```python
from build123d import *

# Parameters (mm, degrees)
F0_W     = 22.5599961265
F0_H     = 4
F1_DEPTH = 150
F2_R     = 2
F3_DEPTH = 9.20100235
F4_SIZE  = 1


# Not quite as in the source:
# - a fillet or chamfer that OpenCascade refuses, or shapes differently, is made with other operations: its cross-section is extruded or revolved along the edge and cut away or added


with BuildPart() as f1:
    # F0 (on Top) → F1 (new body)
    with BuildSketch(Plane.XY):
        Polygon((0, -4), (0, 0), (-8.7200025445, -5.20000235), (-20.5118006432, -5.20000235), (-27.4400038735, -9.20000235), (-8.7200025445, -9.20000235), align=None)
        with Locations((11.2799980633, -2)):
            Rectangle(F0_W, F0_H)
        with Locations((33.8399941898, -2)):
            Rectangle(F0_W, F0_H)
        Polygon((53.8399947975, -5.20000235), (45.119992253, 0), (45.119992253, -4), (53.8399947975, -9.20000235), (72.5599961265, -9.20000235), (65.6317928962, -5.20000235), align=None)
    extrude(amount=F1_DEPTH)

    # F2 (on face) → F3 (cut, through all)
    with BuildSketch(Plane.XZ.offset(9.20000235)):
        with Locations((-14.9400038735, 140)):
            Circle(F2_R)
        with Locations((60.0599961265, 140)):
            Circle(F2_R)
        with Locations((-14.9400038735, 10)):
            Circle(F2_R)
        with Locations((60.0599961265, 10)):
            Circle(F2_R)
    extrude(amount=-F3_DEPTH, mode=Mode.SUBTRACT)

    # F4
    f4_edges = [f1.edges().sort_by_distance(p)[0] for p in [
        (58.059996, -5.200002, 140),
    ]]
    chamfer(f4_edges, length=F4_SIZE)

    # F5: chamfer of 2 on 1 edges, made by hand

    # F5_s1 → F5_t2 (revolve, cut)
    with BuildSketch(Plane.XY.offset(140)):
        Polygon((63.4742096889, -4.7857887876), (62.0599961265, -8.20000235), (62.0599961265, -6.20000235), align=None)
    revolve(axis=Axis((60.0599961265, -6.20000235, 140), (0, -1, 0)), mode=Mode.SUBTRACT)

    # F6: chamfer of 1.5 on 4 edges, made by hand

    # F6_s1 → F6_t2 (revolve, cut)
    with BuildSketch(Plane.XY.offset(10)):
        Polygon((63.5599961265, -5.20000235), (62.0599961265, -6.70000235), (62.0599961265, -5.20000235), align=None)
    revolve(axis=Axis((60.0599961265, -5.20000235, 10), (0, -1, 0)), mode=Mode.SUBTRACT)

    # F6_s3 → F6_t4 (revolve, cut)
    with BuildSketch(Plane.XY.offset(10)):
        Polygon((-11.4400038735, -5.20000235), (-12.9400038735, -6.70000235), (-12.9400038735, -5.20000235), align=None)
    revolve(axis=Axis((-14.9400038735, -5.20000235, 10), (0, -1, 0)), mode=Mode.SUBTRACT)

    # F6_s5 → F6_t6 (revolve, cut)
    with BuildSketch(Plane.XY.offset(140)):
        Polygon((-11.4400038735, -5.20000235), (-12.9400038735, -6.70000235), (-12.9400038735, -5.20000235), align=None)
    revolve(axis=Axis((-14.9400038735, -5.20000235, 140), (0, -1, 0)), mode=Mode.SUBTRACT)

    # F6_s7 → F6_t8 (revolve, cut)
    with BuildSketch(Plane.XY.offset(140)):
        Polygon((62.1741768278, -7.9243457525), (62.0599961265, -8.498370901), (62.0599961265, -8.20000235), align=None)
    revolve(axis=Axis((60.0599961265, -8.20000235, 140), (0, -1, 0)), mode=Mode.SUBTRACT)


solid = f1.part
```
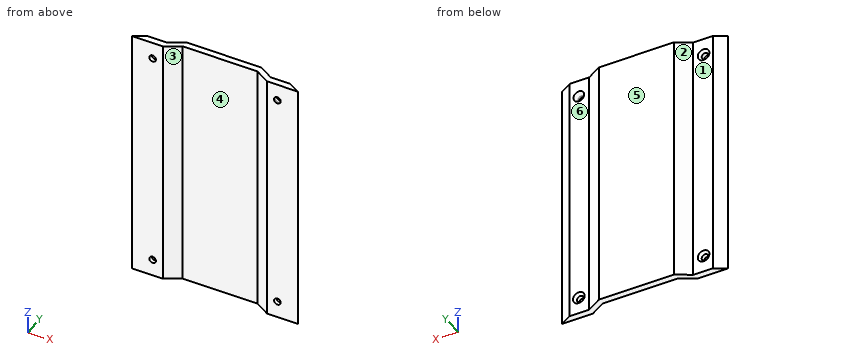
Check sheet for the modelled part. Datum: model origin and axes. Units: mm. Face numbers are marked on the shaded views. A direction names the side the tool comes from. Round coordinates to 2 decimals unless told otherwise and drop trailing zeros. Order: outer loops, then holes, each group sorted by start corner. A loop starts at its lowest first (then second) coordinate and runs counter-clockwise, first axis right, second up.
1) Section check C-C (x = 36). Record the boundary of the cut face in (y, z).
2) Scan lines: line 1 (Y direction, x = 59.5, z = 46); line 2 (Y direction, x = 6, z = 125); line 3 (Z direction, x = 59, y = -6.25). Record each from-to range of solid material in increasing order.
3) Mould release check, pull along X, two halves, no side actions. Record for the marked faces 1, 2, 3 and 4: +X half, -X half, draft (parallel to the pull), parting line (faces both ways), or undercut.
4) Go/stop test with flat-tipped pins: pin 1 Ø3 at (x, z) = (60.06, 140) entering from -Y (3 decimals); pin 2 Ø3.5 at (x, z) = (62, 49) entering from +Y; pin 3 Ø4 at (x, z) = (38, 64.5) entering from -Y. Record where each tip stops, or that it passes through.
5) Section check B-B (z = 24). Record the boundary of the cut face in (x, y), and give its area (3 significant figures).
6) Section check A-A (z = 140). Record the boundary of the cut face in (x, y).
7) Tool access check on the marked faces 5 and 6. Record the directions out of +Z, -Z, +X, -X, +Y, -Y that give a thin tool (end or side, any length) a straight path to the whole face; none if there is none.
Result:
1. outline: (-4, 0) - (0, 0) - (0, 150) - (-4, 150) - close
2. line 1: y = -9.2 to -5.2
2. line 2: y = -4 to 0
2. line 3: z = 0 to 7.79, 12.21 to 137.4, 142.6 to 150
3. face 1: draft
3. face 2: -X half
3. face 3: undercut
3. face 4: undercut
4. pin 1: passes through
4. pin 2: stops at y = -5.2
4. pin 3: stops at y = -4
5. outline: (-27.44, -9.2) - (-8.72, -9.2) - (0, -4) - (45.12, -4) - (53.84, -9.2) - (72.56, -9.2) - (65.63, -5.2) - (53.84, -5.2) - (45.12, 0) - (0, 0) - (-8.72, -5.2) - (-20.51, -5.2) - close
5. area: 372 mm2
6. outline: (-27.44, -9.2) - (-16.94, -9.2) - (-16.94, -6.7) - (-18.44, -5.2) - (-20.51, -5.2) - close; (-12.94, -9.2) - (-8.72, -9.2) - (0, -4) - (45.12, -4) - (53.84, -9.2) - (58.06, -9.2) - (58.06, -8.5) - (57.95, -7.92) - (56.82, -5.2) - (53.84, -5.2) - (45.12, 0) - (0, 0) - (-8.72, -5.2) - (-11.44, -5.2) - (-12.94, -6.7) - close; (62.06, -9.2) - (72.56, -9.2) - (65.63, -5.2) - (63.3, -5.2) - (62.17, -7.92) - (62.06, -8.5) - close
7. face 5: +Z, -Z, +X, -X, +Y
7. face 6: +Z, -Z, +X, +Y
